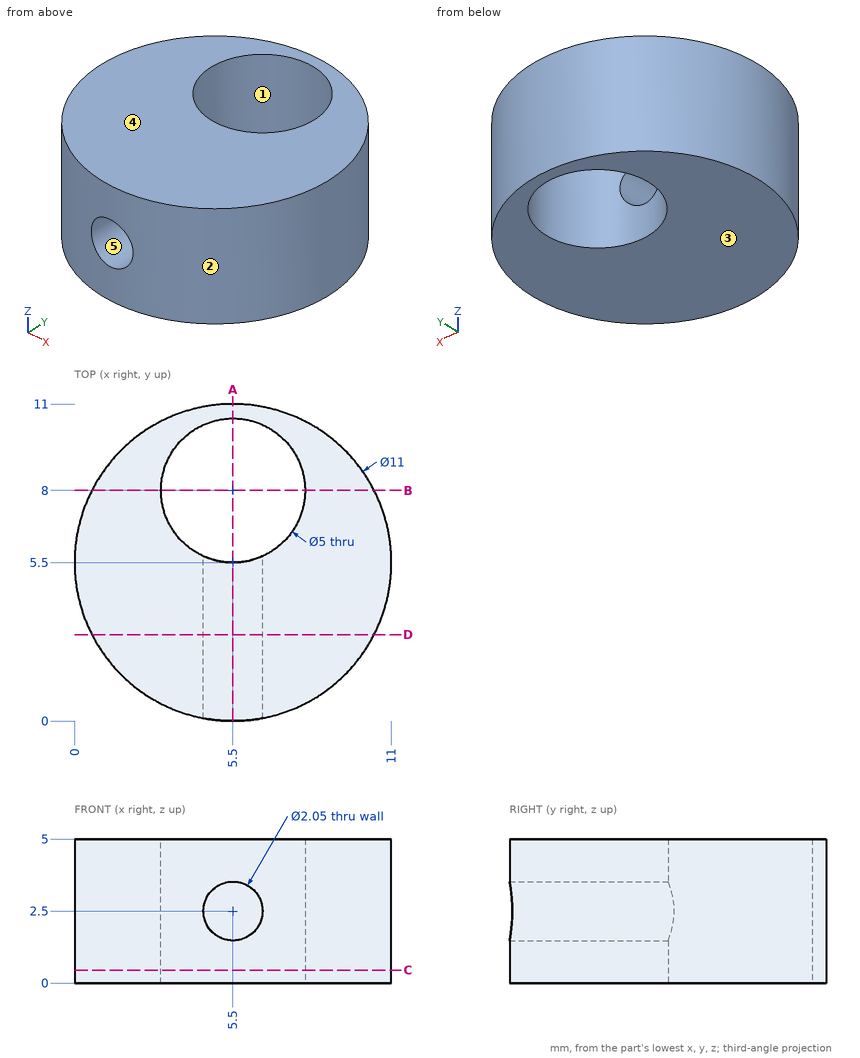
Here's the drawing with two shaded views (mm, measured from the low corner). I have some questions. A direction names the side the tool comes from. Coordinates: 2 decimals unless noted, no trailing zeros. Write each loop counter-clockwise with the first axis right and the second up, starting at its lowest first coordinate (ties: lowest second). Pieces come first, ordered by that corner, then holes. Notation, with made-up numbers: M 24,56 L 41,56 A17 cw 41,80 Z; hole C 3,55.25 d8. An arc over 180 degrees is marked long. Answer as CSV lines item,"result". Start each with the question number.
1) I want a section at A-A, the plane x = 5.5. Please give me the cut outline in (y, z) (3 decimals), and give its area (3 significant figures).
2) For the marked faces 4 and 5, which set-ups out of +Z, -Z, +X, -X, +Y, -Y let a thin tool reach every point of the face, with its end or its side?
3) I want a section at B-B, the plane y = 8. Please give me the cut outline in (x, z).
4) I want a section at D-D, the plane y = 3. Please give me the cut outline in (x, z) (3 decimals), and give its area (3 significant figures).
5) I want a section at C-C, the plane z = 0.45. Please give me the cut outline in (x, y), and give its area (3 significant figures).
6) We'd pull the mould along X, two halves only. Please class the marked faces 1, 2 and 3: +X half, -X half, draft (parallel to the pull), parting line (faces both ways), or undercut.
7) For P1, Ø1, axis at x = 2.5, z = 1.5, coming from the +Y side; P2, Ø6.5, axis at x = 5.5, y = 8, coming from the -Z side; P3, Ø1, axis at y = 7, z = 2.5, coming from the -X side; P4, Ø1.6, axis at x = 5.5, z = 2.5, coming from the -Y side, each with a flat end and sliding along its axis, tell me the tip position at first contact or that it passes through.
8) Please list where these lines run through material, in increasing order: line 1 (Y direction, x = 5.5, z = 3.65); line 2 (Z direction, x = 5.5, y = 3.1) (3 decimals); line 3 (Y direction, x = 5.5, z = 2.65). Write a range as from..to.
Data:
1,outline,"M 0,0 L 5.5,0 L 5.5,1.475 L 0,1.475 Z; M 0,3.525 L 5.5,3.525 L 5.5,5 L 0,5 Z; M 10.5,0 L 11,0 L 11,5 L 10.5,5 Z"
1,area,"18.7 mm^2"
2,face 4,"+Z, +X, -X, +Y, -Y"
2,face 5,"-Y"
3,outline,"M 0.6,0 L 3,0 L 3,5 L 0.6,5 Z; M 8,0 L 10.4,0 L 10.4,5 L 8,5 Z"
4,outline,"M 0.601,0 L 10.399,0 L 10.399,5 L 0.601,5 Z; hole C 5.5,2.5 d2.05"
4,area,"45.7 mm^2"
5,outline,"C 5.5,5.5 d11; hole C 5.5,8 d5"
5,area,"75.4 mm^2"
6,face 1,"undercut"
6,face 2,"parting line"
6,face 3,"draft"
7,P1,"stops at y = 10.4"
7,P2,"stops at z = 0"
7,P3,"stops at x = 0.09"
7,P4,"stops at y = 10.37"
8,line 1,"y = 0..5.5, 10.5..11"
8,line 2,"z = 0..1.475, 3.525..5"
8,line 3,"y = 10.5..11"
